For this review, use the dimensioned drawing (mm, ordinates from the lowest corner) and the shaded views. A direction names the side the tool comes from. Round coordinates to 2 decimals unless told otherwise and drop trailing zeros. Write each loop counter-clockwise with the first axis right and the second up, starting at its lowest first coordinate (ties: lowest second). Pieces come first, ordered by that corner, then holes. Notation, with made-up numbers: (-2.75, 27.25) -> (28.25, 27.25) arc R36 cw to (28.25, 65.25) -> close; hole circle Ø8 at (57.5, -38). An arc over 180 degrees is marked (long way). Answer in a Markdown table with one row per item. Add a question column.
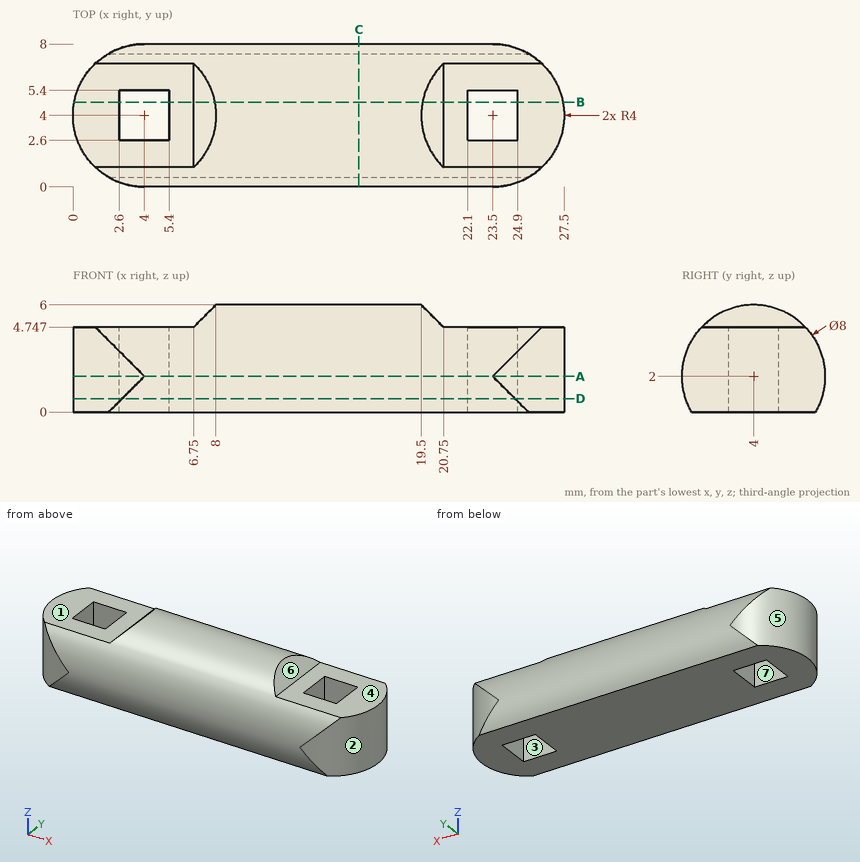
1. We need section C-C (x = 16). Write out the cut boundary in (y, z).
2. We need section B-B (y = 4.75). Write out the cut boundary in (x, z).
3. Tool access review of the marked faces 1, 2, 3 and 4: name each direction out of +Z, -Z, +X, -X, +Y, -Y from which nothing blocks a thin tool from reaching the whole face with its end or side.
4. We need section A-A (z = 2). Write out the cut boundary in (x, y), plus the area to 3 significant figures.
5. Clearance check with flat-ended pins moving along their axes: pin 1 Ø0.8 at (x, z) = (4.5, 1.5) entering from -Y; pin 2 Ø1.7 at (x, y) = (24, 4.5) entering from +Z; pin 3 Ø1 at (y, z) = (4, 5.5) entering from +X; pin 4 Ø3 at (x, z) = (14, 4.5) entering from +Y. State where each tip first meets the part, or that it passes through.
6. For L1, parallel to X at y = 5, z = 1.25; L2, parallel to X at y = 3.5, z = 3.5; L3, parallel to Z at x = 1.75, y = 2.75, list the stretches that pass through material, from the lowest coordinate up. Write a range as [from, to].
7. We need section D-D (z = 0.75). Write out the cut boundary in (x, y), plus the area to 3 significant figures.
8. The part is to be moulded in two halves that separate along Y. For the marked faces 5, 6 and 7, say which applies: pulls with the +Y half, pulls with the -Y half, needs draft (parallel to the pull), parting line crosses it, or undercut.
Response:
| question | item | result |
|---|---|---|
| 1 | outline | (0.54, 0) -> (7.46, 0) arc R4 ccw (long way) to start |
| 2 | outline | (0.07, 0) -> (2.6, 0) -> (2.6, 4.75) -> (0.07, 4.75) -> close; (5.4, 0) -> (22.1, 0) -> (22.1, 4.75) -> (20.75, 4.75) -> (19.57, 5.93) -> (7.93, 5.93) -> (6.75, 4.75) -> (5.4, 4.75) -> close; (24.9, 0) -> (27.43, 0) -> (27.43, 4.75) -> (24.9, 4.75) -> close |
| 3 | face 1 | +Z, -X, +Y, -Y |
| 3 | face 2 | +Z, -Z, +X |
| 3 | face 3 | +Z, -Z |
| 3 | face 4 | +Z, +X, +Y, -Y |
| 4 | outline | (4, 0) -> (23.5, 0) arc R4 ccw to (23.5, 8) -> (4, 8) arc R4 ccw to start; hole (2.6, 2.6) -> (5.4, 2.6) -> (5.4, 5.4) -> (2.6, 5.4) -> close; hole (22.1, 2.6) -> (24.9, 2.6) -> (24.9, 5.4) -> (22.1, 5.4) -> close |
| 4 | area | 191 mm2 |
| 5 | pin 1 | y = 0 |
| 5 | pin 2 | through |
| 5 | pin 3 | x = 20.5 |
| 5 | pin 4 | y = 7.87 |
| 6 | L1 | [0.13, 2.6], [5.4, 22.1], [24.9, 27.37] |
| 6 | L2 | [0.03, 2.6], [5.4, 22.1], [24.9, 27.47] |
| 6 | L3 | [0, 4.75] |
| 7 | outline | (2.75, 0.2) -> (24.75, 0.2) arc R4 ccw to (24.75, 7.8) -> (2.75, 7.8) arc R4 ccw to start; hole (2.6, 2.6) -> (5.4, 2.6) -> (5.4, 5.4) -> (2.6, 5.4) -> close; hole (22.1, 2.6) -> (24.9, 2.6) -> (24.9, 5.4) -> (22.1, 5.4) -> close |
| 7 | area | 182 mm2 |
| 8 | face 5 | parting line crosses it |
| 8 | face 6 | needs draft |
| 8 | face 7 | undercut |
